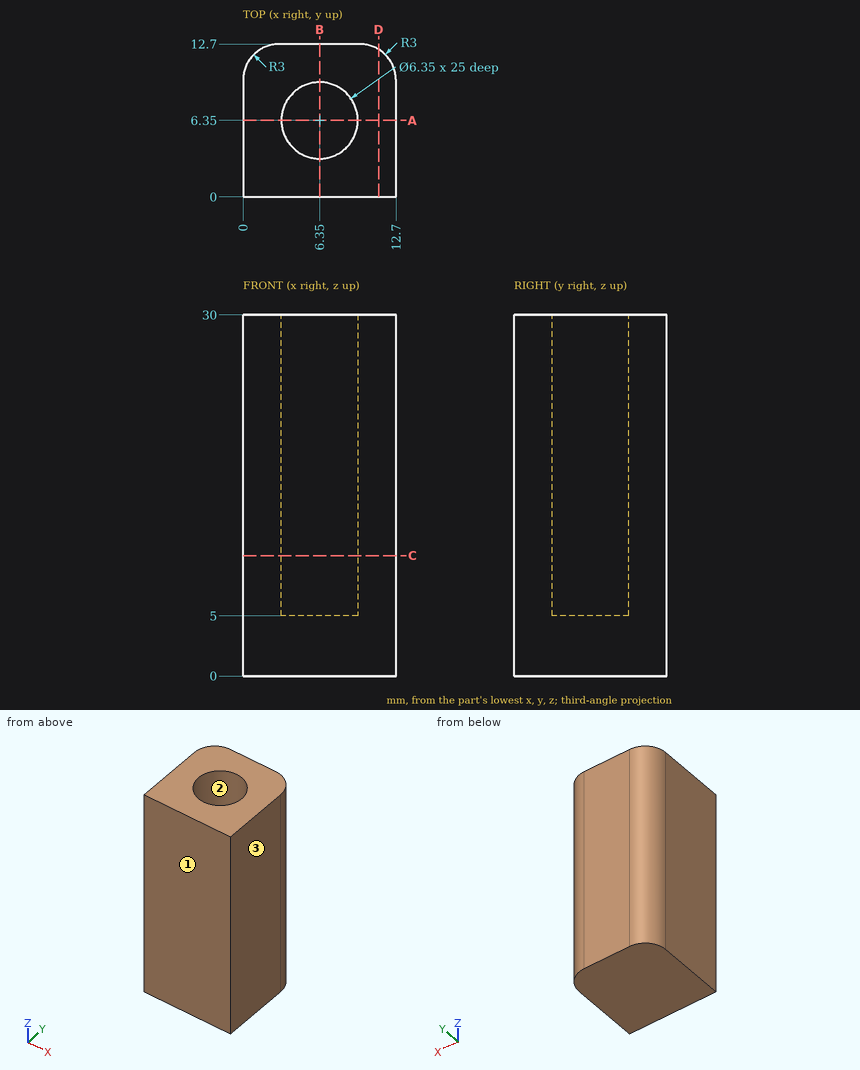
Geometry check sheet. Reference: drawing and pictorial views, mm from the part's lowest x, y, z. Round coordinates to 2 decimals unless told otherwise and drop trailing zeros. Loops run counter-clockwise (first coordinate to the right, second up) from the corner with the lowest first, then second, coordinate; pieces in that order, holes last. Notation, with made-up numbers: M -27.5,38 L 25.5,38 A21 ccw 25.5,66 Z; hole C 62.25,81.25 d5. An arc over 180 degrees is marked long. Return JSON: item names as keys, results as strings. Group by question number.
(1) Scan lines: line 1 along Y through (x, z) = (6.25, 6.5); line 2 along Z through (x, y) = (9, 7); line 3 along Y through (x, z) = (8, 24.5). Record each from-to range of solid material in increasing order. Write a range as [from, to].
(2) Section check C-C, the plane z = 10. Enter the section's corners in (x, y) (3 decimals).
(3) Mould release check, pull along Y, two halves, no side actions. Record for the marked faces 1, 2 and 3: pulls with the +Y half, pulls with the -Y half, needs draft (parallel to the pull), parting line crosses it, or undercut.
(4) Section check D-D, the plane x = 11.25. Enter the section's corners in (y, z).
(5) Section check A-A, the plane y = 6.35. Enter the section's corners in (x, z) (3 decimals).
Data:
{
 "1": {"line 1": "[0, 3.18], [9.52, 12.7]", "line 2": "[0, 5]", "line 3": "[0, 3.64], [9.06, 12.7]"},
 "2": {"outline": "M 0,0 L 12.7,0 L 12.7,9.7 A3 ccw 9.7,12.7 L 3,12.7 A3 ccw 0,9.7 Z; hole C 6.35,6.35 d6.35"},
 "3": {"face 1": "pulls with the -Y half", "face 2": "undercut", "face 3": "needs draft"},
 "4": {"outline": "M 0,0 L 12.27,0 L 12.27,30 L 0,30 Z"},
 "5": {"outline": "M 0,0 L 12.7,0 L 12.7,30 L 9.525,30 L 9.525,5 L 3.175,5 L 3.175,30 L 0,30 Z"}
}
